The listing builds one solid part. Answer for the finished solid, in the listing's coordinates (mm). Face numbers are marked on the shaded views. A direction names the side the tool comes from. Give positions to 0.01 mm unless a question says otherwise; leave off trailing zeros. Loops run counter-clockwise (first coordinate to the right, second up) from the corner with the lowest first, then second, coordinate; pieces in that order, holes last.
Item 1: Consider line 1 along Z through (x, y) = (-5, -39.35); line 2 along Y through (x, z) = (10, 147.75); line 3 along Z through (x, y) = (3.75, -36). Determine where each line is inside the solid, lowest interval first.
Item 2: Each of these flat-tipped pins is pushed along its axis until it touches: pin 1 Ø1 at (x, z) = (5.5, 137.5) entering from +Y; pin 2 Ø4 at (x, y) = (-0.5, -34.5) entering from -Z; pin 3 Ø0.6 at (x, y) = (-10, -33) entering from +Z. Where does it stop, or does it pass through?
Item 3: Section D-D, the plane x = -10 is taken. Give the vertices of the cut face in (y, z).
Item 4: A tool of negligible diameter and unlimited length cuts with its end or side. For the marked faces 1 and 2, from which of +Z, -Z, +X, -X, +Y, -Y can it reach the whole face along a straight path? Write none if from no direction.
Item 5: Section B-B, the plane z = 125 is taken. Give the vertices of the cut face in (x, y).
Item 6: Section C-C, the plane x = -5 is taken. Give the vertices of the cut face in (y, z), and give its area (3 significant figures).
Item 7: Section A-A, the plane x = 0 is taken. Give the vertices of the cut face in (y, z), and give its area (3 significant figures).
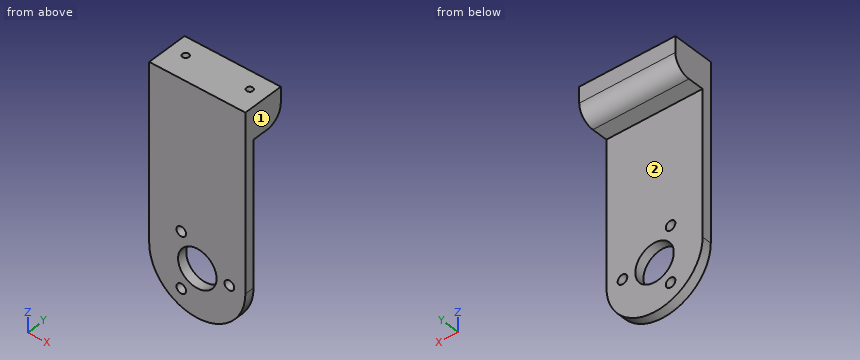
from build123d import *

# Parameters (mm, degrees)
CYLINDER037_R     = 1
CYLINDER037_DEPTH = 8
CYLINDER033_R     = 6
CYLINDER033_DEPTH = 3
CYLINDER034_R     = 1.5
CYLINDER034_DEPTH = 3
ARRAY007_COUNT    = 3
CYLINDER036_R     = 1
CYLINDER036_DEPTH = 8
BOX003_W          = 30
BOX003_H          = 3
BOX003_DEPTH      = 55
BOX005_W          = 30
BOX005_H          = 10
BOX005_DEPTH      = 10
FILLET003_R       = 5
CYLINDER032_R     = 15
CYLINDER032_DEPTH = 3


with BuildPart() as payload_plate_screw002:
    # Cylinder037 → Cylinder037 (new body)
    with BuildSketch(Plane(origin=(-10, -33, 144.7), x_dir=(1, 0, 0), z_dir=(0, 0, 1))):
        Circle(CYLINDER037_R)
    extrude(amount=CYLINDER037_DEPTH)


with BuildPart() as arm_bottom_arc_axis_clearance:
    # Cylinder033 → Cylinder033 (new body)
    with BuildSketch(Plane(origin=(0, -37.5, 97.7), x_dir=(1, 0, 0), z_dir=(0, -1, 0))):
        Circle(CYLINDER033_R)
    extrude(amount=CYLINDER033_DEPTH)


with BuildPart() as arm_screw_holes:
    # Cylinder034 → Cylinder034 (new body)
    with BuildSketch(Plane(origin=(10, -37.5, 97.7), x_dir=(1, 0, 0), z_dir=(0, -1, 0))):
        Circle(CYLINDER034_R)
    extrude(amount=CYLINDER034_DEPTH)

    # Array007: arm-screw-holes ×3 about axis
    array007_axis = Axis((0, 0, 97.7), (0, 1, 0))


with BuildPart() as arm_screw_holes_1:
    add(arm_screw_holes.part)
    for i in range(1, ARRAY007_COUNT):
        add(arm_screw_holes.part.rotate(array007_axis, i * 360 / ARRAY007_COUNT))


with BuildPart() as arm_payload_plate_screw_holes:
    # Cylinder036 → Cylinder036 (new body)
    with BuildSketch(Plane(origin=(10, -33, 144.7), x_dir=(1, 0, 0), z_dir=(0, 0, 1))):
        Circle(CYLINDER036_R)
    extrude(amount=CYLINDER036_DEPTH)

    # Compound: union payload-plate-screw002, arm-bottom-arc-axis-clearance, arm-screw-holes
    add(payload_plate_screw002.part)
    add(arm_bottom_arc_axis_clearance.part)
    add(arm_screw_holes_1.part)


with BuildPart() as arm:
    # Box003 → Box003 (new body)
    with BuildSketch(Plane(origin=(-15, -40.5, 97.7), x_dir=(1, 0, 0), z_dir=(0, 0, 1))):
        with Locations((15, 1.5)):
            Rectangle(BOX003_W, BOX003_H)
    extrude(amount=BOX003_DEPTH)


with BuildPart() as arm_screw_block_with_fillet:
    # Box005 → Box005 (new body)
    with BuildSketch(Plane(origin=(-15, -37.5, 142.7), x_dir=(1, 0, 0), z_dir=(0, 0, 1))):
        with Locations((15, 5)):
            Rectangle(BOX005_W, BOX005_H)
    extrude(amount=BOX005_DEPTH)

    # Fillet003
    fillet003_edges = [arm_screw_block_with_fillet.edges().sort_by_distance(p)[0] for p in [
        (0, -27.5, 142.7),
    ]]
    fillet(fillet003_edges, radius=FILLET003_R)


with BuildPart() as tilt_arm:
    # Cylinder032 → Cylinder032 (new body)
    with BuildSketch(Plane(origin=(0, -37.5, 97.7), x_dir=(1, 0, 0), z_dir=(0, -1, 0))):
        Circle(CYLINDER032_R)
    extrude(amount=CYLINDER032_DEPTH)

    # Fusion015: union arm, arm-screw-block-with-fillet
    add(arm.part)
    add(arm_screw_block_with_fillet.part)

    # Cut026: cut arm-payload-plate-screw-holes
    add(arm_payload_plate_screw_holes.part, mode=Mode.SUBTRACT)


solid = tilt_arm.part
Worked answers:
1. line 1: z = 83.56 to 87.54, 90.54 to 94.38, 101.02 to 104.86, 107.86 to 152.7
1. line 2: y = -40.5 to -34, -32 to -27.5
1. line 3: z = 142.7 to 152.7
2. pin 1: stops at y = -37.5
2. pin 2: stops at z = 142.7
2. pin 3: stops at z = 144.7
3. outline: (-40.5, 86.52) - (-37.5, 86.52) - (-37.5, 142.7) - (-32.5, 142.7) arc R5 ccw to (-27.5, 147.7) - (-27.5, 152.7) - (-32, 152.7) - (-32, 144.7) - (-34, 144.7) - (-34, 152.7) - (-40.5, 152.7) - close
4. face 1: +Z, -Z, +X, +Y, -Y
4. face 2: -Z, +X, -X, +Y
5. outline: (-15, -40.5) - (15, -40.5) - (15, -37.5) - (-15, -37.5) - close
6. outline: (-40.5, 83.56) - (-37.5, 83.56) - (-37.5, 87.54) - (-40.5, 87.54) - close; (-40.5, 90.54) - (-37.5, 90.54) - (-37.5, 94.38) - (-40.5, 94.38) - close; (-40.5, 101.02) - (-37.5, 101.02) - (-37.5, 104.86) - (-40.5, 104.86) - close; (-40.5, 107.86) - (-37.5, 107.86) - (-37.5, 142.7) - (-32.5, 142.7) arc R5 ccw to (-27.5, 147.7) - (-27.5, 152.7) - (-40.5, 152.7) - close
6. area: 264 mm2
7. outline: (-40.5, 82.7) - (-37.5, 82.7) - (-37.5, 91.7) - (-40.5, 91.7) - close; (-40.5, 103.7) - (-37.5, 103.7) - (-37.5, 142.7) - (-32.5, 142.7) arc R5 ccw to (-27.5, 147.7) - (-27.5, 152.7) - (-40.5, 152.7) - close
7. area: 269 mm2
